For this review, use the dimensioned drawing (mm, ordinates from the lowest corner) and the shaded views. A direction names the side the tool comes from. Give positions to 0.01 mm unless a question says otherwise; leave off trailing zeros. Order: outer loops, then holes, each group sorted by start corner. A loop starts at its lowest first (then second) coordinate and runs counter-clockwise, first axis right, second up. Notation, with made-up numbers: M 42.5,26.25 L 91.5,26.25 A19 cw 91.5,56.25 Z; hole C 81,-2 d5. An arc over 180 degrees is marked long. One line per question, with ' | ' between items. Start each with the question number.
1. Insertion check: P1, Ø4, axis at x = 38, z = 12, coming from the -Y side; P2, Ø12, axis at x = 50, y = 12.5, coming from the +Z side. Each pin has a flat end and moves straight along its axis. Give the tip position at first contact, or say it passes through.
2. We need section B-B on y = 14.5. Write out the cut boundary in (x, z), then the cut area to 3 significant figures.
3. Wall thickness on L1, parallel to X at y = 14.5, z = 1.1; L2, parallel to Y at x = 67, z = 19.5; L3, parallel to X at y = 8.25, z = 12.25: over which ranges is each line inside the solid? List them lowest first.
4. For the marked faces 4 and 5, list the 3-axis set-ups (+Z, -Z, +X, -X, +Y, -Y) from which the entire face can be reached by the end or side of a thin tool; tool diameter is ignored.
5. We need section C-C on z = 27. Write out the cut boundary in (x, y), then the cut area to 3 significant figures.
6. We need section D-D on x = 56.5. Write out the cut boundary in (y, z), then the cut area to 3 significant figures.
7. The part is to be moulded in two halves that separate along Y. For the marked faces 1, 2 and 3, say which applies: +Y half, -Y half, draft (parallel to the pull), parting line (faces both ways), or undercut.
8. We need section A-A on x = 12.25. Write out the cut boundary in (y, z).
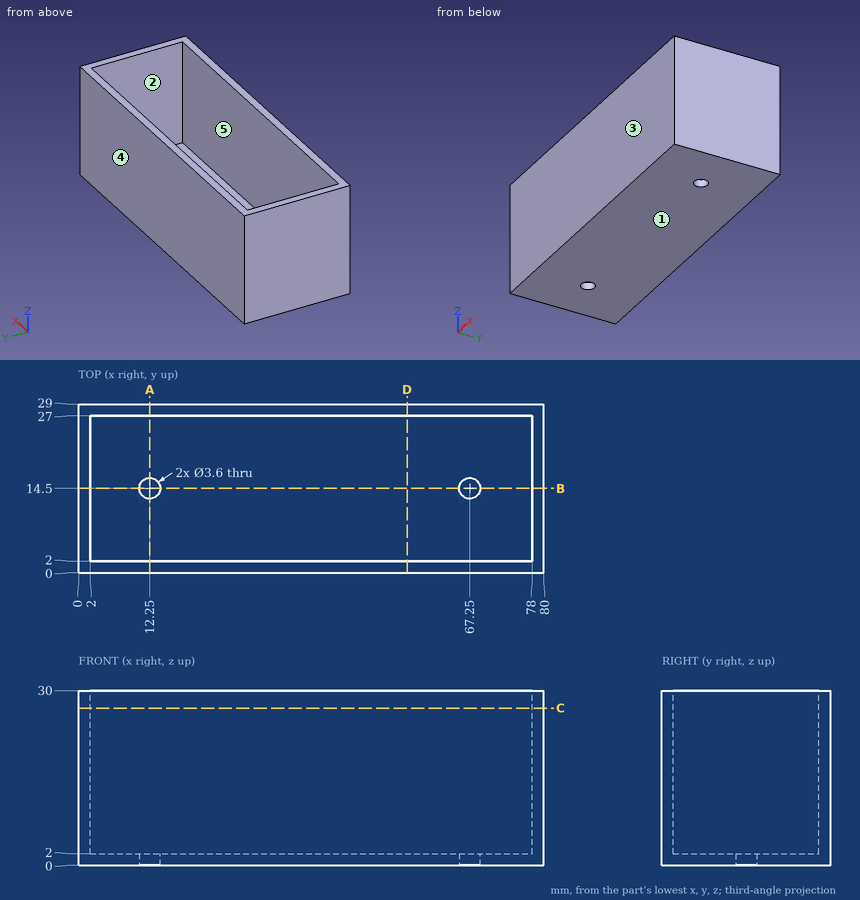
Entries:
1) P1: stops at y = 0 | P2: stops at z = 2
2) outline: M 0,0 L 10.45,0 L 10.45,2 L 2,2 L 2,30 L 0,30 Z; M 14.05,0 L 65.45,0 L 65.45,2 L 14.05,2 Z; M 69.05,0 L 80,0 L 80,30 L 78,30 L 78,2 L 69.05,2 Z | area: 258 mm^2
3) L1: x = 0 to 10.45, 14.05 to 65.45, 69.05 to 80 | L2: y = 0 to 2, 27 to 29 | L3: x = 0 to 2, 78 to 80
4) face 4: +Z, -Z, +X, -X, +Y | face 5: +Z
5) outline: M 0,0 L 80,0 L 80,29 L 0,29 Z; hole M 2,2 L 78,2 L 78,27 L 2,27 Z | area: 420 mm^2
6) outline: M 0,0 L 29,0 L 29,30 L 27,30 L 27,2 L 2,2 L 2,30 L 0,30 Z | area: 170 mm^2
7) face 1: draft | face 2: undercut | face 3: -Y half
8) outline: M 0,0 L 12.7,0 L 12.7,2 L 2,2 L 2,30 L 0,30 Z; M 16.3,0 L 29,0 L 29,30 L 27,30 L 27,2 L 16.3,2 Z
